Input: part model. Units: mm. Frame: model coordinates. Give positions to 0.01 mm unless a question says otherwise; leave off trailing zeros. Loops run counter-clockwise (first coordinate to the right, second up) from the corner with the lowest first, then second, coordinate; pieces in that order, holes last.
from build123d import *

# Parameters (mm, degrees)
F0_W     = 30.6324
F0_H     = 30.6324
F0_W_2   = 24.2824
F0_H_2   = 24.2824
F1_DEPTH = 1.1684
F2_DEPTH = 1.5748


with BuildPart() as f1:
    # F0 (on Top) → F1 (new body)
    with BuildSketch(Plane.XY):
        Rectangle(F0_W, F0_H)
        Rectangle(F0_W_2, F0_H_2, mode=Mode.SUBTRACT)
        Rectangle(F0_W_2, F0_H_2)
    extrude(amount=F1_DEPTH)

    # F0 (on Top) → F2 (join)
    with BuildSketch(Plane.XY):
        Rectangle(F0_W_2, F0_H_2)
    extrude(amount=-F2_DEPTH)


solid = f1.part
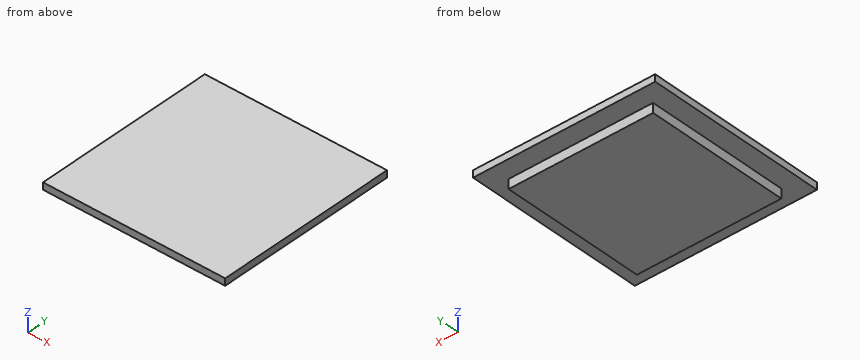
(1) Cut plane C-C (z = -0.9). Return the cut outline in (x, y).
Values follow:
outline: (-12.14, -12.14) - (12.14, -12.14) - (12.14, 12.14) - (-12.14, 12.14) - close
(2) Cut plane A-A (y = 8). Return the cut outline in (x, z), and give its area (3 significant figures).
Values follow:
outline: (-15.32, 0) - (-12.14, 0) - (-12.14, -1.57) - (12.14, -1.57) - (12.14, 0) - (15.32, 0) - (15.32, 1.17) - (-15.32, 1.17) - close
area: 74.0 mm2
(3) Pin query (flat end, axial travel): pin 1 Ø0.8 at (x, z) = (0.5, -1) entering from +Y; pin 2 Ø0.5 at (y, z) = (-0.5, -1) entering from +X; pin 3 Ø1.5 at (x, z) = (-12, -1) entering from -Y. Return the tip coordinate at first contact, or that it passes through.
Values follow:
pin 1: stops at y = 12.14
pin 2: stops at x = 12.14
pin 3: stops at y = -12.14
(4) Ray query, probe 1 along Z at (x, y) = (8, 14); probe 2 along X at (y, z) = (5, -1.25). Return the intervals inside material, ascending.
Values follow:
probe 1: z = 0 to 1.17
probe 2: x = -12.14 to 12.14
